from build123d import *

# Parameters (mm, degrees)
BOSS_EXTRUDE1_DEPTH    = 10
F_8_0MM_DOWEL_HOLE5_D  = 8
F_10_0MM_DOWEL_HOLE1_D = 10


with BuildPart() as part:
    # Sketch1 → Boss-Extrude1 (new body)
    with BuildSketch(Plane.XY):
        Polygon((0, 245.901699437), (75, 245.901699437), (75, 115.901699437), (125, 60), (125, 0), (50, 0), (50, 60), (0, 115.901699437), align=None)
    extrude(amount=BOSS_EXTRUDE1_DEPTH)

    # Ø8.0mm Dowel Hole5 (through all)
    with Locations(Plane.XY.offset(10)):
        with Locations((37.5, 220.901699437), (37.5, 150.901699437)):
            Hole(F_8_0MM_DOWEL_HOLE5_D / 2)

    # Ø10.0mm Dowel Hole1 (through all)
    with Locations(Plane.XY.offset(10)):
        with Locations((37.5, 185.901699437)):
            Hole(F_10_0MM_DOWEL_HOLE1_D / 2)


solid = part.part
CAD build for the part. Positions are in the model's coordinates, mm. A direction names the side the tool comes from. Give positions to 0.01 mm unless a question says otherwise; leave off trailing zeros. Write each loop counter-clockwise with the first axis right and the second up, starting at its lowest first coordinate (ties: lowest second). Pieces come first, ordered by that corner, then holes. Notation, with made-up numbers: (67.5, -5.75) - (103.5, -5.75) arc R11 ccw to (103.5, 5.25) - close; hole circle Ø2 at (-12.75, 73). An arc over 180 degrees is marked (long way). Answer as CSV lines item,"result".
Q1. Flat gauge pins, fed straight in: pin 1 Ø6 at (y, z) = (103.5, 8) entering from +X; pin 2 Ø5 at (y, z) = (108, 3.5) entering from +X; pin 3 Ø6 at (y, z) = (64.5, 3) entering from -X; pin 4 Ø3 at (x, y) = (109, 81.5) entering from -Z. Where does each tip first touch, or does it go through?
Result set:
pin 1,"x = 88.78"
pin 2,"x = 84.3"
pin 3,"x = 43.29"
pin 4,"through"
Q2. Pull direction X, two halves, no side cores. Call faces 4 (the face through (38.021, 224.868, 4.93)), 5 (the face through (125, 30, 5)), 6 (the face through (88, 0, 5)), 7 (the face through (38.58, 181.02, 4.93)): released by +X, released by -X, zero draft, split by the parting line, or undercut.
Result set:
face 4,"undercut"
face 5,"released by +X"
face 6,"zero draft"
face 7,"undercut"
Q3. Drill centre lines: line 1 (Y direction, x = 37.5, z = 6.5); line 2 (Y direction, x = 36, z = 2.5); line 3 (X direction, y = 209, z = 1.5). Where is each one in solid material? Low to high. Write a range as from..to.
Result set:
line 1,"73.98..146.9, 154.9..180.9, 190.9..216.9, 224.9..245.9"
line 2,"75.65..147.19, 154.61..181.13, 190.67..217.19, 224.61..245.9"
line 3,"0..75"
Q4. Band-saw the part on B-B (z = 2.5). Give the cut face in (x, y).
Result set:
outline,"(0, 115.9) - (50, 60) - (50, 0) - (125, 0) - (125, 60) - (75, 115.9) - (75, 245.9) - (0, 245.9) - close; hole circle Ø10 at (37.5, 185.9); hole circle Ø8 at (37.5, 150.9); hole circle Ø8 at (37.5, 220.9)"
Q5. Band-saw the part on D-D (x = 21.5). Give the cut face in (y, z).
Result set:
outline,"(91.86, 0) - (245.9, 0) - (245.9, 10) - (91.86, 10) - close"
Q6. Band-saw the part on C-C (y = 207.5). Give the cut face in (x, z), and give its area (3 significant figures).
Result set:
outline,"(0, 0) - (75, 0) - (75, 10) - (0, 10) - close"
area,"750 mm²"
Q7. 3-axis set-ups, long thin cutter, end or side, ignore diameter. For faces 1 (the face through (35.35, 154.275, 4.93)), 2 (the face through (75, 182, 5)), 3 (the face through (50, 30, 5)): which of +Z, -Z, +X, -X, +Y, -Y reach the whole face in a straight line?
Result set:
face 1,"+Z, -Z"
face 2,"+Z, -Z, +X, +Y"
face 3,"+Z, -Z, -X, -Y"
Q8. Band-saw the part on A-A (x = 37.5). Give the cut face in (y, z), and give its area (3 significant figures).
Result set:
outline,"(73.98, 0) - (146.9, 0) - (146.9, 10) - (73.98, 10) - close; (154.9, 0) - (180.9, 0) - (180.9, 10) - (154.9, 10) - close; (190.9, 0) - (216.9, 0) - (216.9, 10) - (190.9, 10) - close; (224.9, 0) - (245.9, 0) - (245.9, 10) - (224.9, 10) - close"
area,"1,460 mm²"
